Can you work these out from the model? Positions are in its coordinate system, mm. A direction names the side the tool comes from. Coordinates: 2 decimals unless noted, no trailing zeros. Write each loop counter-clockwise with the first axis right and the second up, starting at its lowest first coordinate (ties: lowest second). Pieces come first, ordered by that corner, then holes. Notation, with made-up numbers: (75, 10) -> (124, 10) arc R20 cw to (124, 34) -> close; hole circle Ø4 at (10.5, 59.25). An arc over 180 degrees is marked (long way). Answer as CSV lines item,"result". Start each with the question number.
```python
from build123d import *

# Parameters (mm, degrees)
SKETCH1_R           = 40
SKETCH1_R_2         = 30
BOSS_EXTRUDE1_DEPTH = 100


with BuildPart() as part:
    # Sketch1 → Boss-Extrude1 (new body)
    with BuildSketch(Plane(origin=(0, 0, 0), x_dir=(1, 0, 0), z_dir=(0, 1, 0))):
        Polygon((0, 0), (100, 0), (100, 50), (180, 50), (180, 0), (330, 0), (330, 100), (480, 100), (480, 250), (330, 250), (330, 200), (100, 200), (100, 250), (0, 250), align=None)
        with Locations(Location((215, 120, 0), (0, 0, 90))):
            Circle(SKETCH1_R, mode=Mode.SUBTRACT)
        with Locations(Location((405, 175, 0), (0, 0, 90))):
            Circle(SKETCH1_R_2, mode=Mode.SUBTRACT)
    extrude(amount=BOSS_EXTRUDE1_DEPTH)


solid = part.part
```
Q1. Imagine slicing it at D-D (x = 268). Write out the boundary of the cut face in (y, z), then the cut area to 3 significant figures.
Q2. Imagine slicing it at A-A (x = 405). Write out the boundary of the cut face in (y, z).
Q3. For pin 1 (10 mm diameter, centred on x = 370.5, y = 41, fed in from +Z); pin 2 (25 mm diameter, centred on y = 52.5, z = -33, fed in from +X), each with a flat end and sliding along its axis, tell me the tip position at first contact or that it passes through.
Q4. Which directions (+Z, -Z, +X, -X, +Y, -Y) give clear straight access to the entire face, cutting with the end or side of a thin tool? Please do faces 1 (the face through (139, 49, -50)), 2 (the face through (404, 49, -100)), 3 (the face through (100, 49, -225)).
Q5. Imagine slicing it at B-B (z = -120). Write out the boundary of the cut face in (x, y), then the cut area to 3 significant figures.
Q6. Imagine slicing it at C-C (y = 17.5). Write out the boundary of the cut face in (x, z).
Q7. I need wall thicknesses on L1, parallel to Z at x = 215, y = 70.5; L2, parallel to X at y = 65, z = -175; L3, parallel to Z at x = 405, y = 27. Which ranges of each line are inside material? Lowest first, please.
Q8. If we mould it in two halves opening along X, with no side actions, what happens to faces 4 (the face through (431.615, 49.3, -188.843)), 5 (the face through (183, 100, -155)), 6 (the face through (480, 49, -174)), 7 (the face through (0, 49, -127))? For each: released by +X, released by -X, zero draft, split by the parting line, or undercut.
Entries:
1,outline,"(0, -200) -> (100, -200) -> (100, 0) -> (0, 0) -> close"
1,area,"20,000 mm2"
2,outline,"(0, -250) -> (100, -250) -> (100, -205) -> (0, -205) -> close; (0, -145) -> (100, -145) -> (100, -100) -> (0, -100) -> close"
3,pin 1,"z = -100"
3,pin 2,"x = 330"
4,face 1,"+Z, +Y, -Y"
4,face 2,"+Z, +X, +Y, -Y"
4,face 3,"-Z, +Y, -Y"
5,outline,"(0, 0) -> (175, 0) -> (175, 100) -> (0, 100) -> close; (255, 0) -> (480, 0) -> (480, 100) -> (255, 100) -> close"
5,area,"40,000 mm2"
6,outline,"(0, -250) -> (100, -250) -> (100, -200) -> (330, -200) -> (330, -250) -> (480, -250) -> (480, -100) -> (330, -100) -> (330, 0) -> (180, 0) -> (180, -50) -> (100, -50) -> (100, 0) -> (0, 0) -> close; hole circle Ø80 at (215, -120); hole circle Ø60 at (405, -175)"
7,L1,"-200 to -160, -80 to 0"
7,L2,"0 to 375, 435 to 480"
7,L3,"-250 to -205, -145 to -100"
8,face 4,"undercut"
8,face 5,"zero draft"
8,face 6,"released by +X"
8,face 7,"released by -X"
